CAD build for the part. Positions are in the model's coordinates, mm. A direction names the side the tool comes from. Coordinates: 2 decimals unless noted, no trailing zeros. Order: outer loops, then holes, each group sorted by start corner. A loop starts at its lowest first (then second) coordinate and runs counter-clockwise, first axis right, second up. Notation, with made-up numbers: (17, 71) - (49, 71) arc R15 ccw to (49, 77) - close; hole circle Ø4 at (24, -35.5). An arc over 180 degrees is marked (long way). Return JSON: item names as keys, results as strings.
from build123d import *

# Parameters (mm, degrees)
SKETCH2_R          = 1.25
CUT_EXTRUDE1_DEPTH = 7.649812027


with BuildPart() as part:
    # Sketch1 → Revolve1 (revolve)
    with BuildSketch(Plane.XY, mode=Mode.PRIVATE) as revolve1_sk:
        Polygon((0, 0), (-2.3, 0), (-2.3, 1.6), (-2.075, 1.6), (-2.075, 2.2), (-2.3, 2.2), (-2.3, 3.8), (-1.875, 4.225), (-1.875, 4.8), (-1.95, 4.8), (-1.95, 5.8), (0, 5.8), align=None)
    revolve(revolve1_sk.sketch.rotate(Axis((0, -65.63361976, 0), (0, 1, 0)), 180), axis=Axis((0, -65.63361976, 0), (0, 1, 0)))

    # Sketch2 → Cut-Extrude1 (cut, through all)
    with BuildSketch(Plane(origin=(0, 5.8, 0), x_dir=(1, 0, 0), z_dir=(0, 1, 0))):
        with Locations(Location((0, 0, 0), (0, 0, 180))):
            Circle(SKETCH2_R)
    extrude(amount=-CUT_EXTRUDE1_DEPTH, mode=Mode.SUBTRACT)


solid = part.part
Item 1: Drop flat-ended pins along their axis: P1, Ø1, axis at y = 2.5, z = 1, coming from the +X side (3 decimals); P2, Ø1.5, axis at x = 0.5, y = 3, coming from the -Z side; P3, Ø1, axis at x = 1, y = 1, coming from the -Z side (3 decimals); P4, Ø1, axis at y = 2, z = -1.5, coming from the +X side. Give the stop position or say it passes through.
Findings below:
{"P1": "stops at x = 2.245", "P2": "stops at z = -2.3", "P3": "stops at z = -2.245", "P4": "stops at x = 2.05"}
Item 2: Band-saw the part on A-A, the plane x = 0. List the corners of the cut face in (y, z) (3 decimals), then the cut area to 3 significant figures.
Findings below:
{"outline": "(0, -2.3) - (1.6, -2.3) - (1.6, -2.075) - (2.2, -2.075) - (2.2, -2.3) - (3.8, -2.3) - (4.225, -1.875) - (4.8, -1.875) - (4.8, -1.95) - (5.8, -1.95) - (5.8, -1.25) - (0, -1.25) - close; (0, 1.25) - (5.8, 1.25) - (5.8, 1.95) - (4.8, 1.95) - (4.8, 1.875) - (4.225, 1.875) - (3.8, 2.3) - (2.2, 2.3) - (2.2, 2.075) - (1.6, 2.075) - (1.6, 2.3) - (0, 2.3) - close", "area": "10.5 mm²"}
Item 3: Band-saw the part on B-B, the plane z = 0. List the corners of the cut face in (x, y) (3 decimals), then the cut area to 3 significant figures.
Findings below:
{"outline": "(-2.3, 0) - (-1.25, 0) - (-1.25, 5.8) - (-1.95, 5.8) - (-1.95, 4.8) - (-1.875, 4.8) - (-1.875, 4.225) - (-2.3, 3.8) - (-2.3, 2.2) - (-2.075, 2.2) - (-2.075, 1.6) - (-2.3, 1.6) - close; (1.25, 0) - (2.3, 0) - (2.3, 1.6) - (2.075, 1.6) - (2.075, 2.2) - (2.3, 2.2) - (2.3, 3.8) - (1.875, 4.225) - (1.875, 4.8) - (1.95, 4.8) - (1.95, 5.8) - (1.25, 5.8) - close", "area": "10.5 mm²"}
Item 4: Band-saw the part on D-D, the plane y = 4.6. List the corners of the cut face in (x, z) (3 decimals).
Findings below:
{"outline": "circle Ø3.75 at (0, 0); hole circle Ø2.5 at (0, 0)"}
Item 5: Wall check: L1, parallel to Z at x = 0, y = 1.5; L2, parallel to X at y = 4.15, z = -0.3; L3, parallel to X at y = 2.7, z = -0.6. Give the ranges that are in metal, low to high. Write a range as [from, to].
Findings below:
{"L1": "z = [-2.3, -1.25], [1.25, 2.3]", "L2": "x = [-1.93, -1.21], [1.21, 1.93]", "L3": "x = [-2.22, -1.1], [1.1, 2.22]"}
Item 6: Band-saw the part on C-C, the plane y = 5.4. List the corners of the cut face in (x, z), then the cut area to 3 significant figures.
Findings below:
{"outline": "circle Ø3.9 at (0, 0); hole circle Ø2.5 at (0, 0)", "area": "7.04 mm²"}
Item 7: Mould opens along Z. For faces 1 (the flat face through (-1, 5.8, -1)), 2 (the cylindrical face through (-1.825, 0.811, 1.4)), 3 (the cylindrical face through (1.25, 2.94, 0.05)) say: released by +Z, released by -Z, zero draft, split by the parting line, or undercut.
Findings below:
{"face 1": "zero draft", "face 2": "split by the parting line", "face 3": "undercut"}
Item 8: Which spindle directions (+Z, -Z, +X, -X, +Y, -Y) get a long thin tool onto all of the face, cutting with end or side? Do faces 4 (the cylindrical face through (-1.437, 5.307, -1.318)), 5 (the flat face through (-1, 0, 1)), 6 (the cylindrical face through (1.01, 4.52, -1.58)). Say none if no direction does.
Findings below:
{"face 4": "+Y", "face 5": "+Z, -Z, +X, -X, -Y", "face 6": "none"}
